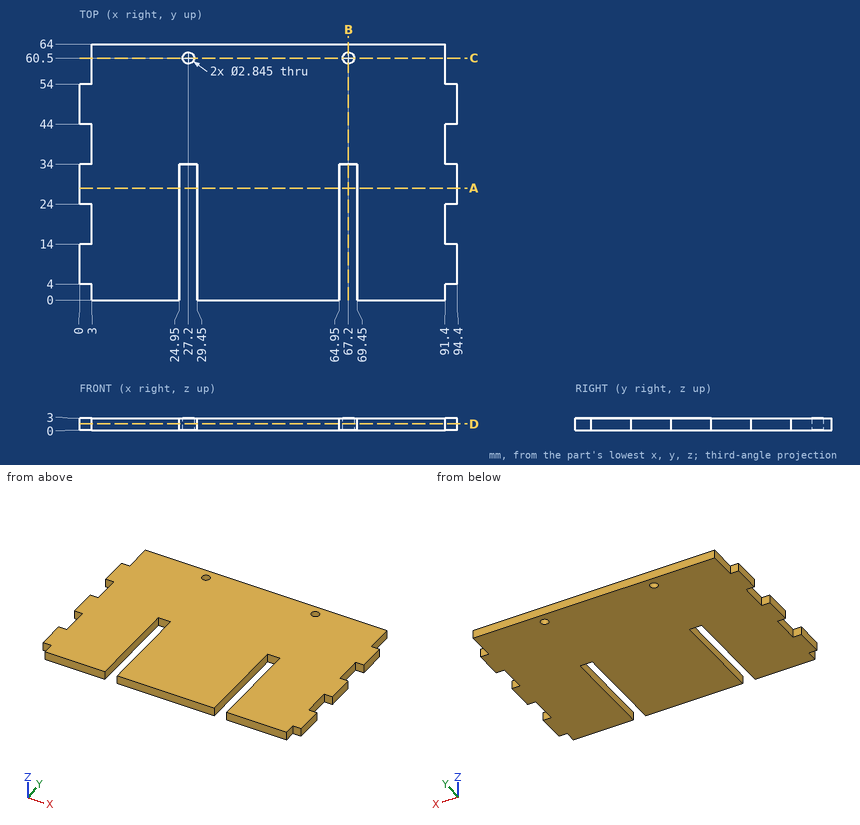
Check sheet for the drawn part. Datum: minimum x, y, z corner. Units: mm. Coordinates: 2 decimals unless noted, no trailing zeros. Loops run counter-clockwise (first coordinate to the right, second up) from the corner with the lowest first, then second, coordinate; pieces in that order, holes last. Notation, with made-up numbers: (56.5, 56.25) -> (71.5, 56.25) arc R18 cw to (71.5, 83.25) -> close; hole circle Ø10 at (32, 66.5). An arc over 180 degrees is marked (long way). Answer in a Markdown table with one row per item.
1) Section check B-B (x = 67.2). Record the cut outline in (y, z).
The answers:
| item | result |
|---|---|
| outline | (34, 0) -> (59.08, 0) -> (59.08, 3) -> (34, 3) -> close; (61.92, 0) -> (64, 0) -> (64, 3) -> (61.92, 3) -> close |
2) Section check C-C (y = 60.5). Record the cut outline in (x, z), and give its area (3 significant figures).
The answers:
| item | result |
|---|---|
| outline | (3, 0) -> (25.78, 0) -> (25.78, 3) -> (3, 3) -> close; (28.62, 0) -> (65.78, 0) -> (65.78, 3) -> (28.62, 3) -> close; (68.62, 0) -> (91.4, 0) -> (91.4, 3) -> (68.62, 3) -> close |
| area | 248 mm2 |
3) Scan lines: line 1 along X through (y, z) = (24.5, 2.4); line 2 along Y through (x, z) = (67.2, 1.1); line 3 along X through (y, z) = (57.5, 0.25). Record each from-to range of solid material in increasing order. Write a range as from..to.
The answers:
| item | result |
|---|---|
| line 1 | x = 0..24.95, 29.45..64.95, 69.45..94.4 |
| line 2 | y = 34..59.08, 61.92..64 |
| line 3 | x = 3..91.4 |
4) Section check A-A (y = 28). Record the cut outline in (x, z), and give its area (3 significant figures).
The answers:
| item | result |
|---|---|
| outline | (0, 0) -> (24.95, 0) -> (24.95, 3) -> (0, 3) -> close; (29.45, 0) -> (64.95, 0) -> (64.95, 3) -> (29.45, 3) -> close; (69.45, 0) -> (94.4, 0) -> (94.4, 3) -> (69.45, 3) -> close |
| area | 256 mm2 |
5) Section check D-D (z = 1.6). Give the number of separate pieces and of enclosed holes in the cut face, and give its area (3 significant figures).
The answers:
| item | result |
|---|---|
| separate pieces | 1 |
| enclosed holes | 2 |
| area | 5,520 mm2 |
6) Depth check by flat-ended pin: P1, Ø1.5, axis at y = 59, z = 1, coming from the +X side; P2, Ø1, axis at x = 26.5, z = 0.5, coming from the -Y side; P3, Ø1.5, axis at x = 93, z = 2, coming from the -Y side. Enter the tip coordinate at first touch or a pass-through.
The answers:
| item | result |
|---|---|
| P1 | stops at x = 91.4 |
| P2 | stops at y = 34 |
| P3 | stops at y = 4 |
